For this review, use the dimensioned drawing (mm, ordinates from the lowest corner) and the shaded views. Round coordinates to 2 decimals unless told otherwise and drop trailing zeros. Write each loop counter-clockwise with the first axis right and the second up, starting at its lowest first coordinate (ties: lowest second). Pieces come first, ordered by that corner, then holes. Notation, with made-up numbers: M 42,64.25 L 55,64.25 A33 cw 55,95.25 Z; hole C 13.25,64.25 d7. An arc over 180 degrees is marked long. Use one line per item in the form item = value. Start each with the question number.
Item 1: Add section B-B (y = 100). State the section outline as (x, z) points (3 decimals), and give its area (3 significant figures).
Item 2: Add section C-C (y = 50). State the section outline as (x, z) points.
Item 3: Add section A-A (x = 50). State the section outline as (y, z) points.
Item 4: For line 1 (X direction, y = 69.5, z = 1.15), list the stretches that pass through material, from the lowest coordinate up. Write a range as [from, to].
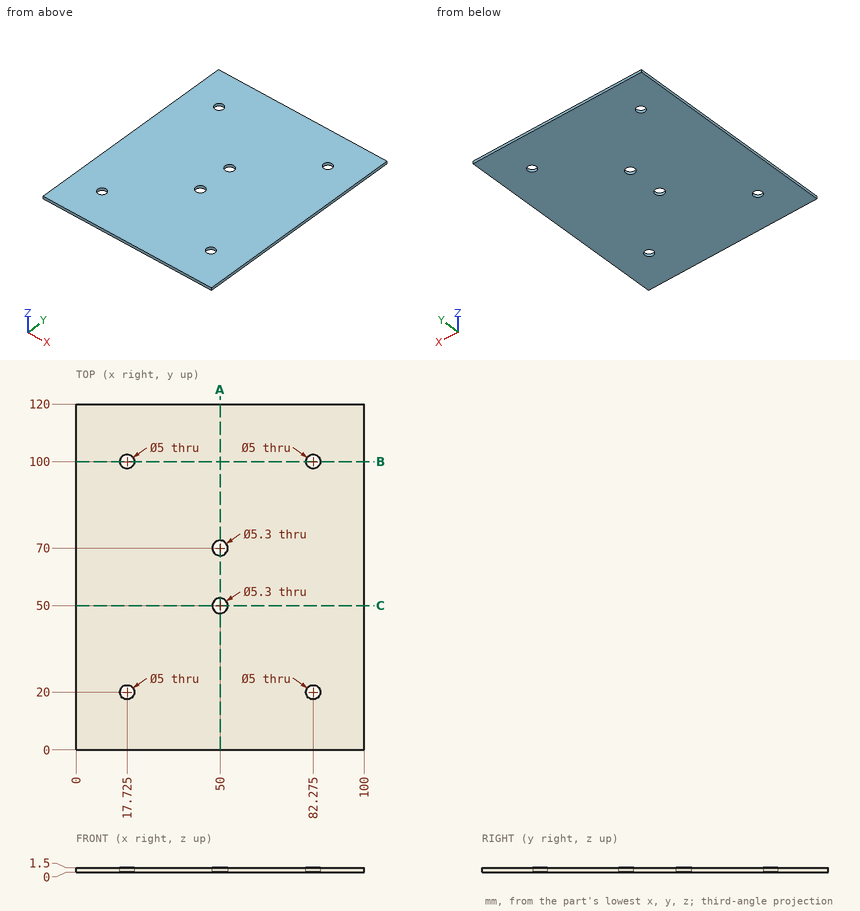
Calculated:
q1.outline = M 0,0 L 15.225,0 L 15.225,1.5 L 0,1.5 Z; M 20.225,0 L 79.775,0 L 79.775,1.5 L 20.225,1.5 Z; M 84.775,0 L 100,0 L 100,1.5 L 84.775,1.5 Z
q1.area = 135 mm^2
q2.outline = M 0,0 L 47.35,0 L 47.35,1.5 L 0,1.5 Z; M 52.65,0 L 100,0 L 100,1.5 L 52.65,1.5 Z
q3.outline = M 0,0 L 47.35,0 L 47.35,1.5 L 0,1.5 Z; M 52.65,0 L 67.35,0 L 67.35,1.5 L 52.65,1.5 Z; M 72.65,0 L 120,0 L 120,1.5 L 72.65,1.5 Z
q4.line_1 = [0, 47.4], [52.6, 100]
